from build123d import *

# Parameters (mm, degrees)
SKETCH1_W           = 100
SKETCH1_H           = 60
SKETCH1_W_2         = 10
SKETCH1_H_2         = 8
SKETCH1_W_3         = 8
SKETCH1_H_3         = 10
BOSS_EXTRUDE1_DEPTH = 4


with BuildPart() as part:
    # Sketch1 → Boss-Extrude1 (new body)
    with BuildSketch(Plane.XY):
        Rectangle(SKETCH1_W, SKETCH1_H)
        with Locations((-40, 30)):
            Rectangle(SKETCH1_W_2, SKETCH1_H_2)
        with Locations((-20, 30)):
            Rectangle(SKETCH1_W_2, SKETCH1_H_2)
        with Locations((0, 30)):
            Rectangle(SKETCH1_W_2, SKETCH1_H_2)
        with Locations((20, 30)):
            Rectangle(SKETCH1_W_2, SKETCH1_H_2)
        with Locations((40, 30)):
            Rectangle(SKETCH1_W_2, SKETCH1_H_2)
        with Locations((50, 20)):
            Rectangle(SKETCH1_W_3, SKETCH1_H_3)
        with Locations((50, 0)):
            Rectangle(SKETCH1_W_3, SKETCH1_H_3)
        with Locations((50, -20)):
            Rectangle(SKETCH1_W_3, SKETCH1_H_3)
        with Locations((-50, 20)):
            Rectangle(SKETCH1_W_3, SKETCH1_H_3)
        with Locations((-50, 0)):
            Rectangle(SKETCH1_W_3, SKETCH1_H_3)
        with Locations((-50, -20)):
            Rectangle(SKETCH1_W_3, SKETCH1_H_3)
    extrude(amount=BOSS_EXTRUDE1_DEPTH)


solid = part.part
For this review, take the finished solid that the model builds, in its own axes (mm). A direction names the side the tool comes from. Round coordinates to 2 decimals unless told otherwise and drop trailing zeros. Write each loop counter-clockwise with the first axis right and the second up, starting at its lowest first coordinate (ties: lowest second). Pieces come first, ordered by that corner, then holes. Notation, with made-up numbers: (12, 72.25) - (32, 72.25) arc R29 cw to (32, 103.25) - close; hole circle Ø9 at (83.25, 33). An arc over 180 degrees is marked (long way). Use a Markdown table: item, result.
Q1. Machinability: for faces 1 (the flat face through (52, 15, 2)), 2 (the flat face through (52, -25, 2)), 3 (the flat face through (25, 32, 2)), which of the approach directions +Z, -Z, +X, -X, +Y, -Y give a long, thin tool a straight path to every point of the face, cutting with its end or side? Answer none if there is none.
Derived:
| item | result |
|---|---|
| face 1 | +Z, -Z, +X |
| face 2 | +Z, -Z, +X, -Y |
| face 3 | +Z, -Z, +Y |
Q2. We need section A-A (x = 30). Give the boundary of the cut face in (y, z).
Derived:
| item | result |
|---|---|
| outline | (-30, 0) - (30, 0) - (30, 4) - (-30, 4) - close |
Q3. Clearance check with flat-ended pins moving along their axes: pin 1 (2 mm diameter, centred on y = 32.5, z = 2.5, fed in from -X); pin 2 (1.5 mm diameter, centred on x = -1.5, y = 14.5, fed in from -Z); pin 3 (1.5 mm diameter, centred on x = 12, z = 1, fed in from +Y); pin 4 (1.2 mm diameter, centred on y = 10.5, z = 2, fed in from +X). State where each tip first meets the part, or that it passes through.
Derived:
| item | result |
|---|---|
| pin 1 | stops at x = -45 |
| pin 2 | stops at z = 0 |
| pin 3 | stops at y = 30 |
| pin 4 | stops at x = 50 |
Q4. We need section B-B (y = 7.5). Give the boundary of the cut face in (x, z), plus the area to 3 significant figures.
Derived:
| item | result |
|---|---|
| outline | (-50, 0) - (50, 0) - (50, 4) - (-50, 4) - close |
| area | 400 mm2 |
Q5. The part is to be moulded in two halves that separate along X. For faces 4 (the flat face through (-35, 32, 2)), 5 (the flat face through (50, -10, 2)), 6 (the flat face through (-50, -28, 2)), 7 (the flat face through (-1, 2, 0)), say which applies: pulls with the +X half, pulls with the -X half, needs draft (parallel to the pull), parting line crosses it, or undercut.
Derived:
| item | result |
|---|---|
| face 4 | undercut |
| face 5 | pulls with the +X half |
| face 6 | pulls with the -X half |
| face 7 | needs draft |
Q6. Wall thickness on line 1 along X through (y, z) = (30.5, 1.4); line 2 along X through (y, z) = (-7.5, 1.1); line 3 along Y through (x, z) = (48.5, 3.2): over which ranges is each line inside the solid? List them lowest first.
Derived:
| item | result |
|---|---|
| line 1 | x = -45 to -35, -25 to -15, -5 to 5, 15 to 25, 35 to 45 |
| line 2 | x = -50 to 50 |
| line 3 | y = -30 to 30 |
